Build history of the part. All positions in model axes, mm. Face numbers are marked on the shaded views. A direction names the side the tool comes from. Coordinates: 2 decimals unless noted, no trailing zeros. Write each loop counter-clockwise with the first axis right and the second up, starting at its lowest first coordinate (ties: lowest second). Pieces come first, ordered by that corner, then holes. Notation, with made-up numbers: (-39, 84) -> (-21, 84) arc R21 ccw to (-21, 96) -> close; hole circle Ø7 at (48.5, 37.25). An arc over 180 degrees is marked (long way). Write each question's results on one line, items separated by ' | '. Start each with the question number.
Q1. Drop flat-ended pins along their axis: pin 1 Ø0.5 at (x, y) = (-2, -5) entering from +Z; pin 2 Ø6 at (y, z) = (-10.5, -5) entering from -X; pin 3 Ø3 at (y, z) = (5, 10.5) entering from +X. Give the stop position or say it passes through.
Q2. Saw through at C-C on z = -9. Give the cut face in (x, y) (3 decimals), and give its area (3 significant figures).
Q3. Saw through at A-A on x = 0. Give the cut face in (y, z) (3 decimals), and give its area (3 significant figures).
Q4. Two-plate mould, pull along X, no slides. Class the marked faces 4, 5 and 6: released by +X, released by -X, zero draft, split by the parting line, or undercut.
Q5. Saw through at D-D on y = -3.5. Give the cut face in (x, z), and give its area (3 significant figures).
Q6. Tool access for the marked faces 1, 2 and 3: list every direction of +Z, -Z, +X, -X, +Y, -Y with a clear straight run to the whole face (end or side of a thin tool).
Q7. Saw through at B-B on y = 6. Give the cut face in (x, z).
Q8. Drill centre lines: line 1 (Z direction, x = 0, y = -8.5); line 2 (X direction, y = 6.25, z = 3.5); line 3 (X direction, y = -10.25, z = 0). Where is each one in solid material? Low to high.
Autodesk Inventor part; units mm, degrees
ref_plane "YZ Plane" through (0, 0, 0) normal (1, 0, 0) x (0, 1, 0)
ref_plane "XZ Plane" through (0, 0, 0) normal (0, 1, 0) x (-1, 0, 0)
ref_plane "XY Plane" through (0, 0, 0) normal (0, 0, 1) x (1, 0, 0)
sketch "Valve Handle" plane through (0, 0, 0) normal (0, 0, 1) x (1, 0, 0)
  line L0 (-2.032, 23.7871) -> (2.032, 23.7871)
  line L1 (-2.032, -23.7871) -> (2.032, -23.7871)
  line L2 (-2.032, 23.7871) -> (-2.032, -23.7871)
  line L3 (2.032, 23.7871) -> (2.032, -23.7871)
  line L4 (0, 11.176) -> (0, -22.606)
  line L5 (0, 11.176) -> (0, -22.606)
  point P0 (0, -1.7145)
  point P1 (0, 0)
  dimension "d146" = 33.782
  dimension "d167" = 11.176
  dimension "d168" = 22.606
sketch "Valve Casing" plane through (0, 0, 0) normal (0, 0, 1) x (1, 0, 0)
  circle A0 centre (0, 0) radius 8.636
  circle A1 centre (0, 0) radius 11.176
  circle A2 centre (0, 0) radius 12.446
  dimension "d149" = 24.892
sketch "Servo Arm Socket" plane through (0, 0, 0) normal (0, 0, 1) x (1, 0, 0)
  arc A0 (4.8166, -0.3016) -> (-4.8166, -0.3016) centre (0, 0) ccw
  line L0 (0, 0) -> (0, -20.32)
  arc A1 (-3.549, -20.5423) -> (3.549, -20.5423) centre (0, -20.32) ccw
  line L1 (-3.549, -20.5423) -> (-4.8166, -0.3016)
  line L2 (4.8166, -0.3016) -> (3.549, -20.5423)
  line L3 (-5.0701, -0.3175) -> (-3.8026, -20.5581)
  arc A2 (-3.8026, -20.5581) -> (3.8026, -20.5581) centre (0, -20.32) ccw
  line L4 (3.8026, -20.5581) -> (5.0701, -0.3175)
  arc A3 (5.0701, -0.3175) -> (-5.0701, -0.3175) centre (0, 0) ccw
  line L5 (-5.0701, -20.6375) -> (-6.3376, -0.3969)
  arc A4 (6.3376, -0.3969) -> (-6.3376, -0.3969) centre (0, 0) ccw
  line L6 (6.3376, -0.3969) -> (5.0701, -20.6375)
  arc A5 (-5.0701, -20.6375) -> (5.0701, -20.6375) centre (0, -20.32) ccw
  dimension "d162" = 9.652
  dimension "d163" = 20.32
  dimension "d164" = 7.112
  dimension "d165" = 0.254
  dimension "d166" = 1.27
sketch "Sketch10" plane through (0, 0, 0) normal (0, 1, 0) x (-1, 0, 0)
  line L0 (0, -14.097) -> (0, 0)
  line L1 (0, 23.7871) -> (0, -23.7871) construction
  line L2 (-2.032, 23.7871) -> (2.032, 23.7871)
  line L3 (-2.032, -23.7871) -> (2.032, -23.7871)
  line L4 (-2.032, 23.7871) -> (-2.032, -23.7871)
  line L5 (2.032, 23.7871) -> (2.032, -23.7871)
  line L6 (0, 11.176) -> (0, -22.606)
  line L7 (0, 11.176) -> (0, -22.606)
  circle A0 centre (0, 0) radius 8.636
  circle A1 centre (0, 0) radius 11.176
  circle A2 centre (0, 0) radius 12.446
  arc A3 (4.8166, -0.3016) -> (-4.8166, -0.3016) centre (0, 0) ccw
  line L8 (0, 0) -> (0, -20.32)
  arc A4 (-3.549, -20.5423) -> (3.549, -20.5423) centre (0, -20.32) ccw
  line L9 (-3.549, -20.5423) -> (-4.8166, -0.3016)
  line L10 (4.8166, -0.3016) -> (3.549, -20.5423)
  line L11 (-5.0701, -0.3175) -> (-3.8026, -20.5581)
  arc A5 (-3.8026, -20.5581) -> (3.8026, -20.5581) centre (0, -20.32) ccw
  line L12 (3.8026, -20.5581) -> (5.0701, -0.3175)
  arc A6 (5.0701, -0.3175) -> (-5.0701, -0.3175) centre (0, 0) ccw
  line L13 (-5.0701, -20.6375) -> (-6.3376, -0.3969)
  arc A7 (6.3376, -0.3969) -> (-6.3376, -0.3969) centre (0, 0) ccw
  line L14 (6.3376, -0.3969) -> (5.0701, -20.6375)
  arc A8 (-5.0701, -20.6375) -> (5.0701, -20.6375) centre (0, -20.32) ccw
  point P0 (2.032, -10.9897)
  point P1 (2.032, -12.279)
  point P2 (-2.032, -12.279)
  point P3 (-2.032, -10.9897)
  point P4 (-2.032, 10.9897)
  point P5 (2.032, 10.9897)
  point P6 (-6.1771, -11.0965)
  point P7 (6.1771, -11.0965)
  point P8 (6.4453, -9.1302)
  point P9 (7.0009, -5.0565)
  point P10 (2.032, 8.3935)
  point P11 (-2.032, 8.3935)
  point P12 (-7.0009, -5.0565)
  point P13 (6.1771, -11.0965)
  point P14 (-6.1771, -11.0965)
  point P15 (2.032, 7.3441)
  point P16 (-7.0009, -5.0565)
  point P17 (7.0009, -5.0565)
  point P18 (6.4453, -9.1302)
  point P19 (2.032, -19.4386)
  point P20 (-6.4453, -9.1302)
  point P21 (2.032, -8.3935)
  point P22 (-2.032, 7.3441)
  point P23 (-2.032, -19.4386)
  point P24 (-2.032, -8.3935)
  point P25 (-5.6686, -11.0802)
  point P26 (5.6686, -11.0802)
  point P27 (5.9718, -6.2385)
  point P28 (-5.9718, -6.2385)
  point P29 (5.7628, -9.5757)
  point P30 (-5.7628, -9.5757)
  point P31 (4.3599, -11.6574)
  point P32 (2.032, -23.5429)
  point P33 (1.5797, -23.7871)
  point P34 (-1.5797, -23.7871)
  point P35 (-2.032, -23.5429)
  point P36 (-4.3599, -11.6574)
extrude "Extrusion21" add sketch "Sketch10" against normal blind 17.145 contours A2 L9 A1 L4 | L5 A1 L10 A2 | A2 L11 A1 L9 | L10 A1 L12 A2 | A2 L13 A1 L11 | L12 A1 L14 A2 | A2 L4 A1 L13 | L14 A1 L5 A2 | A2 L5 A1 L4
extrude "Extrusion22" add sketch "Sketch10" against normal blind 8.128 contours A1 L9 A0 L4 | L5 A0 L10 A1 | A0 L9 A3 L4 | L5 A3 L10 A0 | A1 L11 A0 L9 | L10 A0 L12 A1 | A3 L9 A0 L11 A6 L4 | L5 A6 L12 A0 L10 A3 | A1 L13 A0 L11 | L12 A0 L14 A1 | A6 L11 A0 L13 A7 L4 | L5 A7 L14 A0 L12 A6 | A1 L4 A0 L13 | L14 A0 L5 A1 | A7 L13 A0 L4 | L5 A0 L14 A7
extrude "Extrusion25" add sketch "Sketch10" along normal blind 8.128 contours A5 L3 L4 | L4 L3 A5 L5 L12 A2 L14 A8 L13 L11 | A2 L13 A1 L11 | L5 L3 A5 | L12 A1 L14 A2 | A1 L13 A0 L11 | L12 A0 L14 A1 | A2 L4 A1 L13 | L14 A1 L5 A2 | A6 L4 A7 L6 | L6 A7 L5 A6 | A6 L11 A0 L13 A7 L4 | L5 A7 L14 A0 L12 A6 | A2 L5 A1 L4 | A7 L4 A0 L6 | L6 A0 L5 A7 | A7 L13 A0 L4 | L5 A0 L14 A7 | A1 L6 A0 L4 | L6 A1 L5 A0
sketch "Sketch11" plane through (0, 0, 0) normal (0, 0, 1) x (1, 0, 0)
  point P0 (0, 0)
extrude "Extrusion27" add sketch "Sketch10" against normal blind 10.922 contours L4 L3 A5 L5 L12 A2 L14 A8 L13 L11
properties part number "Servo Adapter 4"
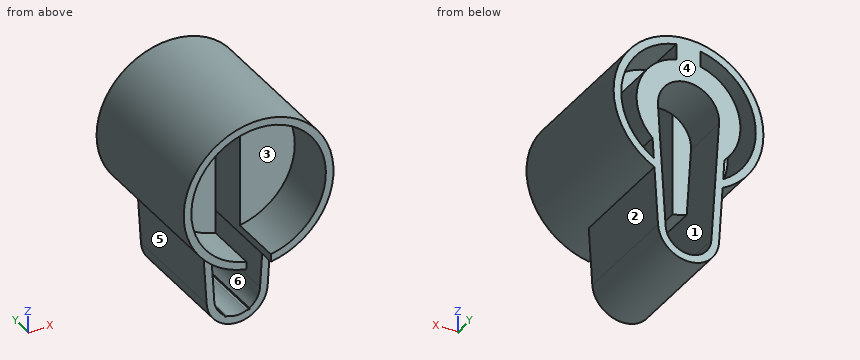
Returned:
1) pin 1: stops at z = 12.32 | pin 2: stops at x = -12.28 | pin 3: stops at x = 8.6
2) outline: (-8.597, -17.145) -> (-6.626, -17.145) -> (-6.626, -8.128) -> (-2.032, -8.128) -> (-2.032, 0) -> (-4.526, 0) -> (-4.526, 8.128) -> (-5.799, 8.128) -> (-5.799, 0) -> (-6.626, 0) -> (-6.626, 8.128) -> (-8.597, 8.128) -> close; (2.032, -8.128) -> (6.626, -8.128) -> (6.626, -17.145) -> (8.597, -17.145) -> (8.597, 8.128) -> (6.626, 8.128) -> (6.626, 0) -> (5.799, 0) -> (5.799, 8.128) -> (4.526, 8.128) -> (4.526, 0) -> (2.032, 0) -> close | area: 195 mm2
3) outline: (-17.145, 11.176) -> (0, 11.176) -> (0, 5.08) -> (8.128, 5.08) -> (8.128, 12.446) -> (-17.145, 12.446) -> close; (-10.922, -25.4) -> (8.128, -25.4) -> (8.128, -24.13) -> (-10.922, -24.13) -> close | area: 106 mm2
4) face 4: zero draft | face 5: released by -X | face 6: undercut
5) outline: (-5.67, -11.08) -> (-5.07, -20.64) arc R5.08 ccw to (5.07, -20.64) -> (5.67, -11.08) arc R12.45 ccw (long way) to start; hole (-4.36, -11.66) -> (-3.8, -20.56) arc R3.81 ccw to (-2.03, -23.54) -> (-2.03, -23.79) -> (-1.58, -23.79) arc R3.81 ccw to (1.58, -23.79) -> (2.03, -23.79) -> (2.03, -23.54) arc R3.81 ccw to (3.8, -20.56) -> (4.36, -11.66) arc R12.45 cw to (2.03, -12.28) -> (2.03, 10.99) arc R11.18 ccw to (-2.03, 10.99) -> (-2.03, -12.28) arc R12.45 cw to start | area: 431 mm2
6) face 1: +Y | face 2: -Z, +X, +Y, -Y | face 3: -Y
7) outline: (-5.67, -11.08) -> (-5.07, -20.64) arc R5.08 ccw to (5.07, -20.64) -> (5.67, -11.08) arc R12.45 ccw (long way) to start; hole (-5.97, -6.24) arc R8.64 cw to (-2.03, 8.39) -> (-2.03, 10.99) arc R11.18 ccw to (-5.76, -9.58) -> close; hole (-5.07, -0.32) -> (-3.8, -20.56) arc R3.81 ccw to (3.8, -20.56) -> (5.07, -0.32) arc R5.08 ccw (long way) to start; hole (2.03, 8.39) arc R8.64 cw to (5.97, -6.24) -> (5.76, -9.58) arc R11.18 ccw to (2.03, 10.99) -> close
8) line 1: z = -25.4 to -24.13, 11.18 to 12.45 | line 2: x = -11.94 to -10.61, -7.89 to -3.68, 3.68 to 7.89, 10.61 to 11.94 | line 3: x = -12.45 to -11.18, 11.18 to 12.45
